from build123d import *

# Parameters (mm, degrees)
EXTRUDE_1_DEPTH     = 90
SKETCH_2_W          = 90
SKETCH_2_H          = 17.75
EXTRUDE_2_DEPTH     = 8.2
SKETCH_3_W          = 90
SKETCH_3_H          = 102.45
EXTRUDE_3_DEPTH     = 8.2
SKETCH_4_W          = 3.95
SKETCH_4_H          = 2.25
CUT_EXTRUDE_1_DEPTH = 171.45954982
SKETCH_5_W          = 3.95
SKETCH_5_H          = 29.5
CUT_EXTRUDE_2_DEPTH = 171.45954982
SKETCH_6_W          = 3.95
SKETCH_6_H          = 9
CUT_EXTRUDE_3_DEPTH = 171.45954982
SKETCH_7_W          = 3.95
SKETCH_7_H          = 29.5
CUT_EXTRUDE_4_DEPTH = 171.45954982
SKETCH_8_W          = 3.95
SKETCH_8_H          = 6.2
CUT_EXTRUDE_5_DEPTH = 171.45954982
SKETCH_9_W          = 2.25
SKETCH_9_H          = 3.95
CUT_EXTRUDE_6_DEPTH = 171.45954982
SKETCH_10_W         = 4.5
SKETCH_10_H         = 3.95
CUT_EXTRUDE_7_DEPTH = 171.45954982
SKETCH_11_W         = 2.25
SKETCH_11_H         = 3.95
CUT_EXTRUDE_8_DEPTH = 171.45954982
SKETCH_12_W         = 19.6
SKETCH_12_H         = 96.1
CUT_EXTRUDE_9_DEPTH = 86.2
EXTRUDE_START       = -90
EXTRUDE_5_DEPTH     = 90
EXTRUDE_6_DEPTH     = 0.2


# Read off the part's stored shape, not the designer's step: Бобышка-Вытянуть5
with BuildPart() as part:
    # Эскиз1 → Бобышка-Вытянуть1 (new body)
    with BuildSketch(Plane(origin=(90, 0, 0), x_dir=(0, 0, -1), z_dir=(1, 0, 0))):
        with BuildLine():
            Line((6.75, 40.906238208), (6.75, 135.75))
            Line((6.75, 135.75), (-11.593761792, 135.75))
            ThreePointArc((-11.593761792, 135.75), (-15.325, 134.5), (-11.593761793, 133.25))
            Line((-11.593761793, 133.25), (-11, 133.25))
            Line((-11, 133.25), (-11, 99.75))
            Line((-11, 99.75), (-11.593761792, 99.75))
            ThreePointArc((-11.593761792, 99.75), (-15.325, 98.5), (-11.593761792, 97.25))
            Line((-11.593761792, 97.25), (-11, 97.25))
            Line((-11, 97.25), (-11, 84.25))
            Line((-11, 84.25), (-11.593761792, 84.25))
            ThreePointArc((-11.593761792, 84.25), (-15.325, 83), (-11.593761792, 81.75))
            Line((-11.593761792, 81.75), (-11, 81.75))
            Line((-11, 81.75), (-11, 48.25))
            Line((-11, 48.25), (-11.593761792, 48.25))
            ThreePointArc((-11.593761792, 48.25), (-15.325, 47), (-11.593761792, 45.75))
            Line((-11.593761792, 45.75), (-11, 45.75))
            Line((-11, 45.75), (-11, 41.5))
            Line((-11, 41.5), (-6.75, 41.5))
            Line((-6.75, 41.5), (-6.75, 40.906238208))
            ThreePointArc((-6.75, 40.906238208), (-5.5, 37.175), (-4.25, 40.906238208))
            Line((-4.25, 40.906238208), (-4.25, 41.5))
            Line((-4.25, 41.5), (4.25, 41.5))
            Line((4.25, 41.5), (4.25, 40.906238208))
            ThreePointArc((4.25, 40.906238208), (5.5, 37.175), (6.75, 40.906238208))
        make_face()
    extrude(amount=-EXTRUDE_1_DEPTH)

    # Эскиз2 → Бобышка-Вытянуть2 (add)
    with BuildSketch(Plane(origin=(0, 135.75, 0), x_dir=(-1, 0, 0), z_dir=(0, 1, 0))):
        with Locations((-45, 2.125)):
            Rectangle(SKETCH_2_W, SKETCH_2_H)
    extrude(amount=EXTRUDE_2_DEPTH)

    # Эскиз3 → Бобышка-Вытянуть3 (add)
    with BuildSketch(Plane(origin=(0, 0, -6.75), x_dir=(-1, 0, 0), z_dir=(0, 0, -1))):
        with Locations((-45, 92.725)):
            Rectangle(SKETCH_3_W, SKETCH_3_H)
    extrude(amount=EXTRUDE_3_DEPTH)

    # Эскиз4 → Вырез-Вытянуть1 (cut, through all)
    with BuildSketch(Plane.ZY):
        with Locations((-12.975, 42.625)):
            Rectangle(SKETCH_4_W, SKETCH_4_H)
    extrude(amount=-CUT_EXTRUDE_1_DEPTH, mode=Mode.SUBTRACT)

    # Эскиз5 → Вырез-Вытянуть2 (cut, through all)
    with BuildSketch(Plane.ZY):
        with Locations((-12.975, 65)):
            Rectangle(SKETCH_5_W, SKETCH_5_H)
    extrude(amount=-CUT_EXTRUDE_2_DEPTH, mode=Mode.SUBTRACT)

    # Эскиз6 → Вырез-Вытянуть3 (cut, through all)
    with BuildSketch(Plane.ZY):
        with Locations((-12.975, 90.75)):
            Rectangle(SKETCH_6_W, SKETCH_6_H)
    extrude(amount=-CUT_EXTRUDE_3_DEPTH, mode=Mode.SUBTRACT)

    # Эскиз7 → Вырез-Вытянуть4 (cut, through all)
    with BuildSketch(Plane.ZY):
        with Locations((-12.975, 116.5)):
            Rectangle(SKETCH_7_W, SKETCH_7_H)
    extrude(amount=-CUT_EXTRUDE_4_DEPTH, mode=Mode.SUBTRACT)

    # Эскиз8 → Вырез-Вытянуть5 (cut, through all)
    with BuildSketch(Plane.ZY):
        with Locations((-12.975, 140.85)):
            Rectangle(SKETCH_8_W, SKETCH_8_H)
    extrude(amount=-CUT_EXTRUDE_5_DEPTH, mode=Mode.SUBTRACT)

    # Эскиз9 → Вырез-Вытянуть6 (cut, through all)
    with BuildSketch(Plane.ZY):
        with Locations((-9.875, 141.975)):
            Rectangle(SKETCH_9_W, SKETCH_9_H)
    extrude(amount=-CUT_EXTRUDE_6_DEPTH, mode=Mode.SUBTRACT)

    # Эскиз10 → Вырез-Вытянуть7 (cut, through all)
    with BuildSketch(Plane.ZY):
        with Locations((0, 141.975)):
            Rectangle(SKETCH_10_W, SKETCH_10_H)
    extrude(amount=-CUT_EXTRUDE_7_DEPTH, mode=Mode.SUBTRACT)

    # Эскиз11 → Вырез-Вытянуть8 (cut, through all)
    with BuildSketch(Plane.ZY):
        with Locations((9.875, 141.975)):
            Rectangle(SKETCH_11_W, SKETCH_11_H)
    extrude(amount=-CUT_EXTRUDE_8_DEPTH, mode=Mode.SUBTRACT)

    # Эскиз12 → Вырез-Вытянуть9 (cut)
    with BuildSketch(Plane(origin=(90, 0, 0), x_dir=(0, 0, -1), z_dir=(1, 0, 0))):
        with Locations((0, 90.75)):
            Rectangle(SKETCH_12_W, SKETCH_12_H)
    extrude(amount=-CUT_EXTRUDE_9_DEPTH, mode=Mode.SUBTRACT)

    # Бобышка-Вытянуть5 outline → Бобышка-Вытянуть5 (cut)
    with BuildSketch(Plane(origin=(90, 0, 0), x_dir=(0, 0, -1), z_dir=(1, 0, 0)).offset(EXTRUDE_START)):
        with BuildLine():
            ThreePointArc((-6.973940297, 143.95), (-5.5, 140), (-4.026059703, 143.95))
            Line((-4.026059703, 143.95), (-6.973940297, 143.95))
        make_face()
        with BuildLine():
            ThreePointArc((4.026059703, 143.95), (5.5, 140), (6.973940297, 143.95))
            Line((6.973940297, 143.95), (4.026059703, 143.95))
        make_face()
        with BuildLine():
            ThreePointArc((14.95, 135.973940297), (11, 134.5), (14.95, 133.026059703))
            Line((14.95, 133.026059703), (14.95, 135.973940297))
        make_face()
        with BuildLine():
            ThreePointArc((14.95, 99.973940297), (11, 98.5), (14.95, 97.026059703))
            Line((14.95, 97.026059703), (14.95, 99.973940297))
        make_face()
        with BuildLine():
            ThreePointArc((14.95, 84.473940297), (11, 83), (14.95, 81.526059703))
            Line((14.95, 81.526059703), (14.95, 84.473940297))
        make_face()
        with BuildLine():
            ThreePointArc((14.95, 48.473940297), (11, 47), (14.95, 45.526059703))
            Line((14.95, 45.526059703), (14.95, 48.473940297))
        make_face()
    extrude(amount=EXTRUDE_5_DEPTH, mode=Mode.SUBTRACT)

    # Эскиз21 → Бобышка-Вытянуть6 (add)
    with BuildSketch(Plane.ZY):
        with BuildLine():
            Line((-14.95, 49.276213414), (-5.5, 37.175))
            ThreePointArc((-5.5, 37.175), (-16.275606707, 38.500606707), (-14.95, 49.276213414))
        make_face()
        with BuildLine():
            Line((5.5, 37.175), (15.252051369, 46.45464203))
            ThreePointArc((15.252051369, 46.45464203), (14.740776792, 37.227868536), (5.5, 37.175))
        make_face()
        with BuildLine():
            Line((-14.95, 132.138029851), (-2.788562926, 143.95))
            ThreePointArc((-2.788562926, 143.95), (-16.483808441, 145.883823994), (-14.95, 132.138029851))
        make_face()
        with BuildLine():
            Line((15.325, 134.5), (3.036005332, 143.95))
            ThreePointArc((3.036005332, 143.95), (15.809128056, 147.845015034), (15.325, 134.5))
        make_face()
    extrude(amount=-EXTRUDE_6_DEPTH)


solid = part.part
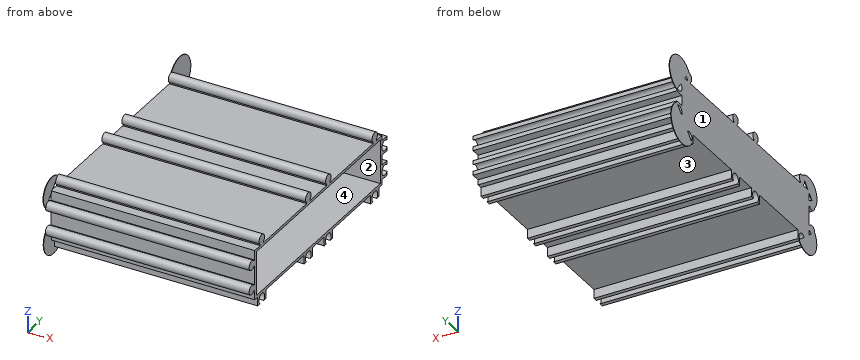
Work out the finished part from the listing and answer in its coordinate system (mm). Face numbers are marked on the shaded views. A direction names the side the tool comes from. Coordinates: 2 decimals unless noted, no trailing zeros. Write each loop counter-clockwise with the first axis right and the second up, starting at its lowest first coordinate (ties: lowest second). Pieces come first, ordered by that corner, then holes. Notation, with made-up numbers: (67, 48) - (115, 48) arc R16 cw to (115, 72) - close; hole circle Ø2 at (18, 54.25). An arc over 180 degrees is marked (long way). One line per question, with ' | ' between items.
1) Find section C-C, the plane z = -13.25. Give the number of separate pieces and of enclosed holes in the cut face, and give its area (3 significant figures).
Checks:
separate pieces: 8 | enclosed holes: 0 | area: 725 mm2
2) Flat-ended cylindrical pins translate along their axes: P1, Ø2, axis at x = 62, y = 43.5, coming from the +Z side; P2, Ø7, axis at y = 134.5, z = -13.25, coming from the -X side; P3, Ø1.2, axis at x = 23.5, z = -12, coming from the -Y side; P4, Ø6, axis at x = 25, y = 132, coming from the -Z side. Find the tip coordinate at first contact, or state that the pin passes through.
Checks:
P1: z = 11 | P2: x = 0 | P3: y = 43.75 | P4: z = -14.95
3) For the marked faces 3 and 4, determine the directions among +Z, -Z, +X, -X, +Y, -Y from which every point of the face is accessible in a straight line to the end or side of a thin tool.
Checks:
face 3: -Z, +X, -X | face 4: +X
4) Consider probe 1 along Z at (x, y) = (59.5, 72.5); probe 2 along Y at (x, z) = (73.5, 8.5); probe 3 along Y at (x, z) = (61.5, 5.5) (3 decimals). Determine where each line is inside the solid, lowest interval first. Write a range as [from, to].
Checks:
probe 1: [-11, -9.8], [9.8, 11] | probe 2: [41.5, 42.7], [138.8, 143.95] | probe 3: [37.175, 42.7], [138.8, 140]
5) The mould has two halves that part along Y. Classify the marked faces 1 and 2: +Y half, -Y half, draft (parallel to the pull), parting line (faces both ways), or undercut.
Checks:
face 1: draft | face 2: undercut
6) Find section A-A, the plane y = 109.5. Determine the outline of the cut face in (x, z), and give its area (3 significant figures).
Checks:
outline: (0, -11) - (90, -11) - (90, -9.8) - (3.8, -9.8) - (3.8, 9.8) - (90, 9.8) - (90, 11) - (0, 11) - close | area: 290 mm2
7) Find section B-B, the plane z = 0. Determine the outline of the cut face in (x, y), and give its area (3 significant figures).
Checks:
outline: (0, 41.5) - (90, 41.5) - (90, 42.7) - (3.8, 42.7) - (3.8, 138.8) - (90, 138.8) - (90, 140) - (0, 140) - close | area: 581 mm2
